from build123d import *

# Parameters (mm, degrees)
PAD005_DEPTH            = 1
SKETCH006_W             = 4
SKETCH006_H             = 4
PAD006_DEPTH            = 12
SKETCH007_R             = 0.45
POCKET_DEPTH            = 10
SKETCH021_W             = 0.35
SKETCH021_H             = 1
POCKET004_DEPTH         = 3
CHAMFER_SIZE            = 1.5
BODY003_PLACEMENT_ANGLE = 90


with BuildPart() as part:
    # Sketch005 → Pad005 (new body)
    with BuildSketch(Plane.XY):
        Polygon((0, -11), (3.5, -7.5), (3.5, 7.5), (0, 11), (-3.5, 7.5), (-3.5, -7.5), align=None)
    extrude(amount=PAD005_DEPTH)

    # Sketch006 (on Face8 of Pad005) → Pad006 (join)
    with BuildSketch(Plane.XY.offset(1)):
        with Locations((0, 6)):
            Rectangle(SKETCH006_W, SKETCH006_H)
    extrude(amount=PAD006_DEPTH)

    # Sketch007 (on Face12 of Pad006) → Pocket (cut)
    with BuildSketch(Plane(origin=(0, 8, 0), x_dir=(-1, 0, 0), z_dir=(0, 1, 0))):
        with Locations((0, 9)):
            Circle(SKETCH007_R)
    extrude(amount=-POCKET_DEPTH, mode=Mode.SUBTRACT)

    # Sketch021 (on Face13 of Pocket) → Pocket004 (cut)
    with BuildSketch(Plane.XY.offset(13)):
        with Locations((0, 4.5)):
            Rectangle(SKETCH021_W, SKETCH021_H)
    extrude(amount=-POCKET004_DEPTH, mode=Mode.SUBTRACT)

    # Chamfer
    chamfer_edges = [part.edges().sort_by_distance(p)[0] for p in [
        (2, 6, 13),
        (-2, 6, 13),
    ]]
    chamfer(chamfer_edges, length=CHAMFER_SIZE)


with BuildPart() as part_1:
    # Body003 placement: moved
    add(part.part.moved(Location((0, 9, 2))).rotate(Axis((0, 9, 2), (1, 0, 0)), BODY003_PLACEMENT_ANGLE))


solid = part_1.part
Geometry: final body of the model. Coordinates: model frame, mm. A direction names the side the tool comes from. Coordinates: 2 decimals unless noted, no trailing zeros. Order: outer loops, then holes, each group sorted by start corner. A loop starts at its lowest first (then second) coordinate and runs counter-clockwise, first axis right, second up.
(1) Section query C-C (y = 2.25). Return the cut outline in (x, z).
(2) Material intervals for probe 1 along Y at (x, z) = (0, 8.55); probe 2 along X at (y, z) = (0, 9.15); probe 3 along Z at (x, y) = (0.25, 7.75), sorted ascending.
(3) Section query B-B (x = -1.25). Return the cut outline in (y, z).
(4) Section query D-D (x = -3). Return the cut outline in (y, z), plus the area to 3 significant figures.
(5) Draft query along X for faces 6 (the face through (0.175, -2.5, 6.5)), 7 (the face through (-0.175, -2.5, 6.5)), 8 (the face through (-1.8, 8.5, -7.2)), 9 (the face through (0, 9, 2)). Return one class per face: pulls with the +X half, pulls with the -X half, needs draft (parallel to the pull), parting line crosses it, or undercut.
(6) Access query for faces 1 (the face through (0, 2, 6)), 2 (the face through (-2, 3, 8)), 3 (the face through (2, 3, 8)), 4 (the face through (1.8, 8.5, 11.2)), 5 (the face through (0, 2, 10)). Directions: +Z, -Z, +X, -X, +Y, -Y. A direction counts if a zero-diameter tool reaches every point of the face in a straight line with its end or side. Return the directions, or none.
(7) Section query A-A (y = -2.75). Return the cut outline in (x, z) (3 decimals), plus the area to 4 significant figures.
(8) First-contact query: pin 1 (1.2 mm diameter, centred on x = -1, y = 0.5, fed in from -Z); pin 2 (2 mm diameter, centred on x = 0.5, z = -2.5, fed in from -Y); pin 3 (1.1 mm diameter, centred on y = -2, z = 6.5, fed in from -X). Flat tips, straight axial feed; report the tip coordinate or a pass-through.
Solution:
1. outline: (-2, 6) - (2, 6) - (2, 10) - (-2, 10) - close
2. probe 1: y = -4 to -0.45, 0.45 to 9
2. probe 2: x = -2 to -0.45, 0.45 to 2
2. probe 3: z = 6 to 10
3. outline: (-3.25, 6) - (8, 6) - (8, -7.75) - (9, -7.75) - (9, 11.75) - (8, 11.75) - (8, 10) - (-3.25, 10) - close
4. outline: (8, -6) - (9, -6) - (9, 10) - (8, 10) - close
4. area: 16.0 mm2
5. face 6: undercut
5. face 7: undercut
5. face 8: pulls with the -X half
5. face 9: needs draft
6. face 1: -Z, +X, -X, -Y
6. face 2: +Z, -Z, -X, -Y
6. face 3: +Z, -Z, +X, -Y
6. face 4: +Z, +X, +Y, -Y
6. face 5: +Z, +X, -X, -Y
7. outline: (-1.75, 6) - (-0.175, 6) - (-0.175, 7) - (0.175, 7) - (0.175, 6) - (1.75, 6) - (1.75, 10) - (-1.75, 10) - close
7. area: 13.65 mm2
8. pin 1: stops at z = 6
8. pin 2: stops at y = 8
8. pin 3: stops at x = -2
